from build123d import *

# Parameters (mm, degrees)
F0_W     = 127
F0_H     = 203.2
F1_DEPTH = 12.7
F3_D     = 6.7564
F4_W     = 76.2
F4_H     = 165.1
F5_DEPTH = 12.7
F7_R     = 12.7
F8_D     = 5.1054
F8_DEPTH = 22.859997
F8_TIP   = 1.5338169022
F9_SIZE2 = 88.9
F9_SIZE  = 25.4
F10_R    = 9.525
F11_R    = 6.35


with BuildPart() as f1:
    # F0 (on Right) → F1 (new body)
    with BuildSketch(Plane.YZ):
        with Locations((63.5, 101.6)):
            Rectangle(F0_W, F0_H)
    extrude(amount=F1_DEPTH)

    # F3 (through all)
    with Locations(Plane.YZ.offset(12.7)):
        with Locations((6.35, 31.75), (50.8, 31.75), (50.8, 6.35), (6.35, 6.35)):
            Hole(F3_D / 2)

    # F4 (on face) → F5 (cut, through all)
    with BuildSketch(Plane.YZ.offset(12.7)):
        with Locations((38.1, 120.65)):
            Rectangle(F4_W, F4_H)
    extrude(amount=-F5_DEPTH, mode=Mode.SUBTRACT)

    # F7
    f7_edges = [f1.edges().sort_by_distance(p)[0] for p in [
        (6.35, 76.2, 38.1),
    ]]
    fillet(f7_edges, radius=F7_R)

    # F8
    with Locations(Plane.XZ.offset(-76.2)):
        with Locations((6.35, 190.5), (6.35, 127), (6.35, 63.5)):
            Hole(F8_D / 2, depth=F8_DEPTH)
            with Locations((0, 0, -(F8_DEPTH + F8_TIP / 2))):  # 118° drill point
                Cone(0, F8_D / 2, F8_TIP, mode=Mode.SUBTRACT)

    # F9
    f9_edges = [f1.edges().sort_by_distance(p)[0] for p in [
        (6.35, 127, 203.2),
    ]]
    f9_side = f1.faces().sort_by_distance((6.35, 101.6, 203.2))[0]
    chamfer(f9_edges, length=F9_SIZE, length2=F9_SIZE2, reference=f9_side)

    # F10
    f10_edges = [f1.edges().sort_by_distance(p)[0] for p in [
        (6.35, 127, 0),
        (6.35, 101.6, 203.2),
        (6.35, 127, 114.3),
    ]]
    fillet(f10_edges, radius=F10_R)

    # F11
    f11_edges = [f1.edges().sort_by_distance(p)[0] for p in [
        (6.35, 0, 38.1),
        (6.35, 0, 0),
    ]]
    fillet(f11_edges, radius=F11_R)


solid = f1.part
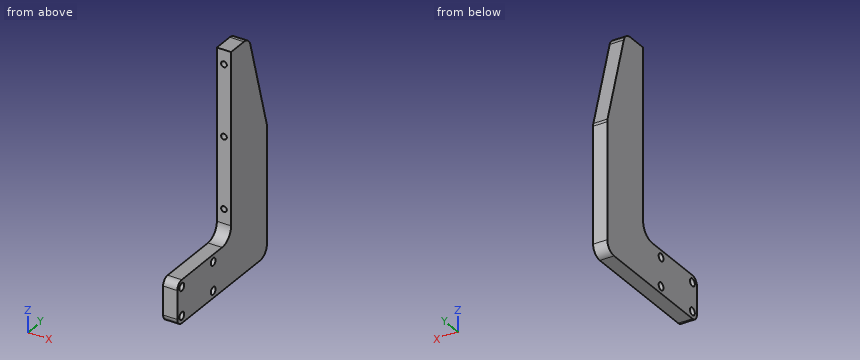
Source: CAD feature listing. Evaluate the final solid. Frame: model axes, mm. Round coordinates to 2 decimals unless told otherwise and drop trailing zeros. Order: outer loops, then holes, each group sorted by start corner. A loop starts at its lowest first (then second) coordinate and runs counter-clockwise, first axis right, second up. Notation, with made-up numbers: (61, 55) - (119, 55) arc R24 cw to (119, 86) - close; hole circle Ø4 at (-20, 19). An arc over 180 degrees is marked (long way). Use a Markdown table: item, result. Add a question column.
1. Section query B-B (z = 157). Return the cut outline in (x, y), then the cut area to 3 significant figures.
2. First-contact query: pin 1 (1 mm diameter, centred on x = 8, z = 112, fed in from -Y); pin 2 (4 mm diameter, centred on x = 6.35, z = 190.5, fed in from -Y); pin 3 (3 mm diameter, centred on x = 9, z = 48, fed in from -Y); pin 4 (6 mm diameter, centred on y = 6.35, z = 6.35, fed in from -X). Flat tips, straight axial feed; report the tip coordinate or a pass-through.
3. Line query: probe 1 along Z at (x, y) = (6.35, 86); probe 2 along Z at (x, y) = (6, 81); probe 3 along Z at (x, y) = (10, 50.8). Output: solid intervals per line, ascending.
4. Section query A-A (y = 21.5). Return the cut outline in (x, z), then the cut area to 3 significant figures.
Derived:
| question | item | result |
|---|---|---|
| 1 | outline | (0, 76.2) - (12.7, 76.2) - (12.7, 114.8) - (0, 114.8) - close |
| 1 | area | 490 mm2 |
| 2 | pin 1 | y = 76.2 |
| 2 | pin 2 | y = 99.39 |
| 2 | pin 3 | y = 75.45 |
| 2 | pin 4 | through |
| 3 | probe 1 | 0 to 60.95, 66.05 to 124.45, 129.55 to 187.95, 193.05 to 203.2 |
| 3 | probe 2 | 0 to 60.97, 66.03 to 124.47, 129.53 to 187.97, 193.03 to 203.2 |
| 3 | probe 3 | 0 to 2.97, 9.73 to 28.37, 35.13 to 38.1 |
| 4 | outline | (0, 0) - (12.7, 0) - (12.7, 38.1) - (0, 38.1) - close |
| 4 | area | 484 mm2 |
